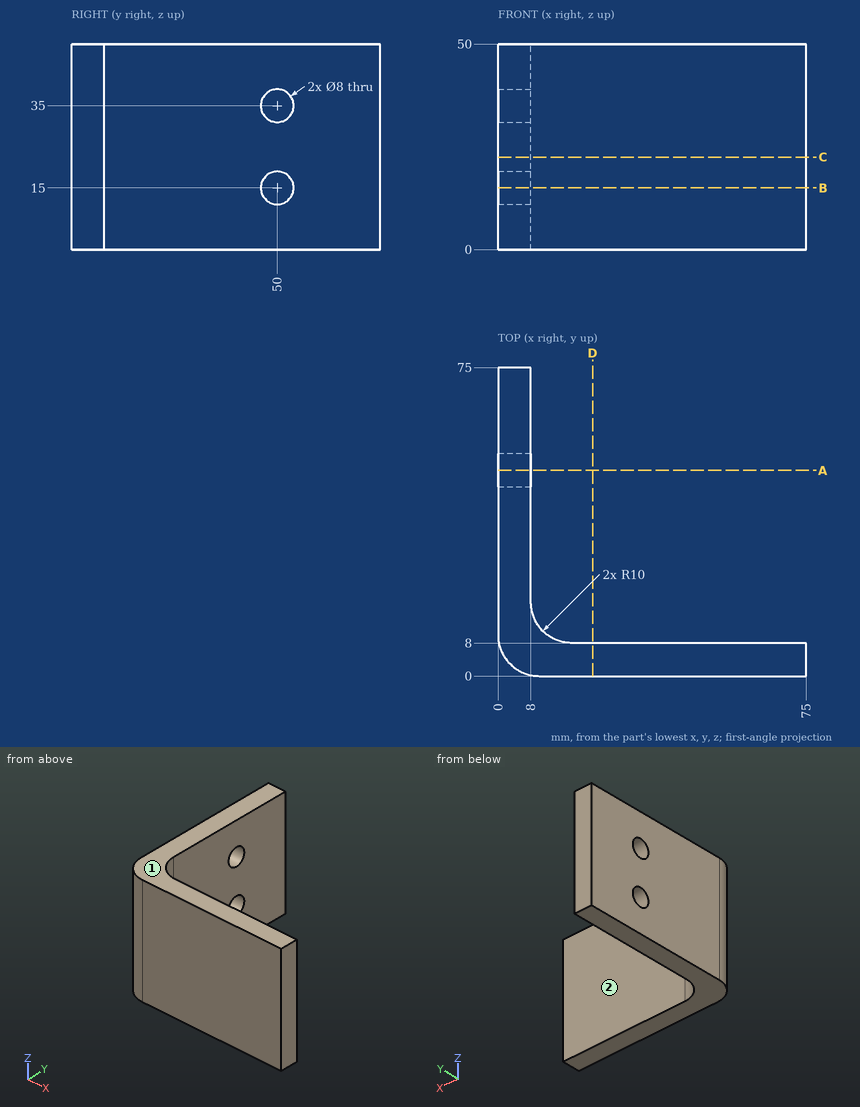
For this review, use the dimensioned drawing (mm, ordinates from the lowest corner) and the shaded views. A direction names the side the tool comes from. Give positions to 0.01 mm unless a question says otherwise; leave off trailing zeros. Loops run counter-clockwise (first coordinate to the right, second up) from the corner with the lowest first, then second, coordinate; pieces in that order, holes last.
Item 1: For line 1 along Z through (x, y) = (4.75, 50); line 2 along Y through (x, z) = (37.5, 27.5), list the stretches that pass through material, from the lowest coordinate up.
Item 2: Take a section at D-D, the plane x = 23. State the section outline as (y, z) points.
Item 3: Take a section at C-C, the plane z = 22.5. State the section outline as (x, y) points, and give its area (3 significant figures).
Item 4: Take a section at B-B, the plane z = 15. State the section outline as (x, y) points, and give its area (3 significant figures).
Item 5: Insertion check: pin 1 (4 mm diameter, centred on y = 37, z = 24, fed in from +X); pin 2 (15 mm diameter, centred on x = 32.5, z = 24.5, fed in from +Y); pin 3 (5 mm diameter, centred on y = 50, z = 35, fed in from -X). Each pin has a flat end and moves straight along its axis. Give the tip position at first contact, or say it passes through.
Item 6: Take a section at A-A, the plane y = 50. State the section outline as (x, z) points.
Item 7: Tool access review of the marked faces 1 and 2: name each direction out of +Z, -Z, +X, -X, +Y, -Y from which nothing blocks a thin tool from reaching the whole face with its end or side.
Calculated:
1. line 1: z = 0 to 11, 19 to 31, 39 to 50
1. line 2: y = 0 to 8
2. outline: (0, 0) - (8, 0) - (8, 50) - (0, 50) - close
3. outline: (0, 10) arc R10 ccw to (10, 0) - (75, 0) - (75, 8) - (18, 8) arc R10 cw to (8, 18) - (8, 75) - (0, 75) - close
3. area: 1,140 mm2
4. outline: (0, 10) arc R10 ccw to (10, 0) - (75, 0) - (75, 8) - (18, 8) arc R10 cw to (8, 18) - (8, 46) - (0, 46) - close; (0, 54) - (8, 54) - (8, 75) - (0, 75) - close
4. area: 1,070 mm2
5. pin 1: stops at x = 8
5. pin 2: stops at y = 8
5. pin 3: passes through
6. outline: (0, 0) - (8, 0) - (8, 11) - (0, 11) - close; (0, 19) - (8, 19) - (8, 31) - (0, 31) - close; (0, 39) - (8, 39) - (8, 50) - (0, 50) - close
7. face 1: +Z, +X, -X, +Y, -Y
7. face 2: +Z, -Z, +X, +Y
